Autodesk Inventor part; units mm, degrees
ref_plane "YZ Plane" through (0, 0, 0) normal (1, 0, 0) x (0, 1, 0)
ref_plane "XZ Plane" through (0, 0, 0) normal (0, 1, 0) x (-1, 0, 0)
ref_plane "XY Plane" through (0, 0, 0) normal (0, 0, 1) x (1, 0, 0)
sketch "Sketch1" plane through (0, 0, 0) normal (0, 0, 1) x (1, 0, 0)
  line L0 (8, 0.0718) -> (2, 3.5359)
  line L1 (2, 3.5359) -> (2, 10.4641)
  line L2 (2, 10.4641) -> (8, 13.9282)
  line L3 (8, 13.9282) -> (14, 10.4641)
  line L4 (14, 10.4641) -> (14, 3.5359)
  line L5 (14, 3.5359) -> (8, 0.0718)
  point P0 (0, 0)
  point P1 (8, 7)
  dimension "d1" = 12
extrude "Extrusion1" add sketch "Sketch1" along normal blind 18
sketch "Sketch2" plane through (0, 0, 0) normal (0, 0, -1) x (-1, 0, 0)
  circle A0 centre (-8, 7) radius 3.1
  point P0 (0, 0)
  dimension "d5" = 6.2
extrude "Extrusion2" cut sketch "Sketch2" against normal blind 14
sketch "Sketch3" plane through (0, 0, 18) normal (0, 0, 1) x (1, 0, 0)
  line L0 (14, 3.5359) -> (8, 0.0718)
  line L1 (14, 3.5359) -> (2, 3.5359)
  line L2 (2, 3.5359) -> (2, 10.4641)
  line L3 (2, 10.4641) -> (14, 10.4641)
  line L4 (14, 10.4641) -> (14, 3.5359)
  point P0 (0, 0)
  dimension "d12" = 6.9282
extrude "Extrusion3" add sketch "Sketch3" along normal blind 17
sketch "Sketch4" plane through (2, 10.4641, 18) normal (0, 1, 0) x (1, 0, 0)
  line L0 (12, 0) -> (12, -17)
  line L1 (12, -17) -> (16, -17)
  line L2 (0, 0) -> (0, -17)
  line L3 (12, 0) -> (12, -17)
  line L4 (0, -17) -> (-4, -17)
  line L5 (0, 0) -> (0, -17)
  line L6 (16, -17) -> (16, -3.1957)
  line L7 (-4, -3.1957) -> (0, 3.2792)
  line L8 (16, -3.1957) -> (12, 3.2792)
  line L9 (12, 18) -> (12, 0)
  line L10 (0, 0) -> (0, 3.2792)
  line L11 (12, 0) -> (12, 3)
  line L12 (-4, -17) -> (-4, -3.1957)
  point P0 (-2, 18)
  dimension "d10" = 4
  dimension "d11" = 4
extrude "Extrusion4" add sketch "Sketch4" against normal blind 6.9282
sketch "Sketch5" plane through (2, 10.4641, 18) normal (0, 1, 0) x (1, 0, 0)
  line L0 (16, -17) -> (16, -17)
  line L1 (0, -17) -> (12, -17)
  line L2 (12, -17) -> (12, -1)
  line L3 (12, -1) -> (0, -1)
  line L4 (0, -1) -> (0, -17)
  point P0 (-2, 18)
  point P1 (-4, -17)
extrude "Extrusion5" cut sketch "Sketch5" against normal through all
sketch "Sketch6" plane through (-2, 10.4641, 21.1957) normal (-1, 0, 0) x (0, 0, 1)
  line L0 (13.8043, 0) -> (13.8043, -6.9282)
  circle A0 centre (7.8043, -3.4641) radius 1.5
  point P0 (-21.1957, -10.4641)
  dimension "d18" = 3
extrude "Extrusion6" cut sketch "Sketch6" against normal through all
properties part number "supportrodv1.2"
Build history of the part. All positions in model axes, mm. A direction names the side the tool comes from. Give positions to 0.01 mm unless a question says otherwise; leave off trailing zeros. Order: outer loops, then holes, each group sorted by start corner. A loop starts at its lowest first (then second) coordinate and runs counter-clockwise, first axis right, second up. Notation, with made-up numbers: M 40.5,35 L 54.5,35 A30 ccw 54.5,66 Z; hole C 5.25,-36 d1. An arc over 180 degrees is marked long. Write item = value, one per line. Start each with the question number.
(1) Slice it at D-D on x = 3.5. Write the cut outline in (y, z), plus the area to 3 significant figures.
(2) Slice it at B-B on y = 7. Write the cut outline in (x, z).
(3) Which spindle directions (+Z, -Z, +X, -X, +Y, -Y) get a long thin tool onto all of the face, cutting with end or side? Do faces 1 (the flat face through (2, 7, 7)), 2 (the flat face through (8, 12, 18)), 3 (the flat face through (14, 7, 7)), 4 (the flat face through (8, 2, 18)), 5 (the flat face through (2, 7, 27)). Say none if no direction does.
(4) Pin check, flat tips, straight feed: pin 1 Ø5 at (y, z) = (7, 29) entering from +X; pin 2 Ø1.7 at (x, y) = (7.5, 11.5) entering from +Z; pin 3 Ø3.5 at (x, y) = (8.5, 8) entering from +Z; pin 4 Ø4 at (y, z) = (10.5, 5) entering from -X. Stop position of each tip, or through.
(5) Slice it at A-A on z = 2.5. Write the cut outline in (x, y).
(6) Two-plate mould, pull along Y, no slides. Class faces 6 (the cylindrical face through (15.97, 7.07, 27.5)), 7 (the flat face through (4.958, 12.172, 8.874)), 8 (the flat face through (11.042, 1.828, 8.874)), 9 (the flat face through (16, 7, 35)): released by +Y, released by -Y, zero draft, split by the parting line, or undercut.
(7) Slice it at C-C on z = 26.5. Write the cut outline in (x, y), plus the area to 3 significant figures.
(8) Probe L1, parallel to Y at x = 15.1, z = 29; L2, parallel to X at y = 4.75, z = 25.5; L3, parallel to Y at x = 0.5, z = 18. List the from-to ranges inside material, lowest first. Write a range as [from, to].
Responses:
q1.outline = M 2.67,0 L 11.33,0 L 11.33,18 L 10.46,18 L 10.46,19 L 3.54,19 L 3.54,18 L 2.67,18 Z
q1.area = 163 mm2
q2.outline = M -2,21.2 L 2,14.72 L 2,0 L 4.9,0 L 4.9,14 L 11.1,14 L 11.1,0 L 14,0 L 14,14.72 L 18,21.2 L 18,27.5 L 14,27.5 L 14,19 L 2,19 L 2,27.5 L -2,27.5 Z; M -2,30.5 L 2,30.5 L 2,35 L -2,35 Z; M 14,30.5 L 18,30.5 L 18,35 L 14,35 Z
q3.face_1 = -Z, -X, +Y, -Y
q3.face_2 = +Z, +X, -X, +Y
q3.face_3 = -Z, +X, +Y, -Y
q3.face_4 = +Z, +X, -X, -Y
q3.face_5 = +Z, +Y, -Y
q4.pin_1 = 18
q4.pin_2 = 18
q4.pin_3 = 19
q4.pin_4 = 2
q5.outline = M 2,3.54 L 8,0.07 L 14,3.54 L 14,10.46 L 8,13.93 L 2,10.46 Z; hole C 8,7 d6.2
q6.face_6 = undercut
q6.face_7 = released by +Y
q6.face_8 = released by -Y
q6.face_9 = zero draft
q7.outline = M -2,3.54 L 2,3.54 L 2,10.46 L -2,10.46 Z; M 14,3.54 L 18,3.54 L 18,10.46 L 14,10.46 Z
q7.area = 55.4 mm2
q8.L1 = [3.54, 5.5], [8.5, 10.46]
q8.L2 = [-2, 2], [14, 18]
q8.L3 = [3.54, 10.46]
